Input: part model. Units: mm. Frame: model coordinates. Face numbers are marked on the shaded views. A direction names the side the tool comes from. Give positions to 0.01 mm unless a question says otherwise; leave off trailing zeros. Loops run counter-clockwise (first coordinate to the right, second up) from the corner with the lowest first, then second, coordinate; pieces in that order, holes last.
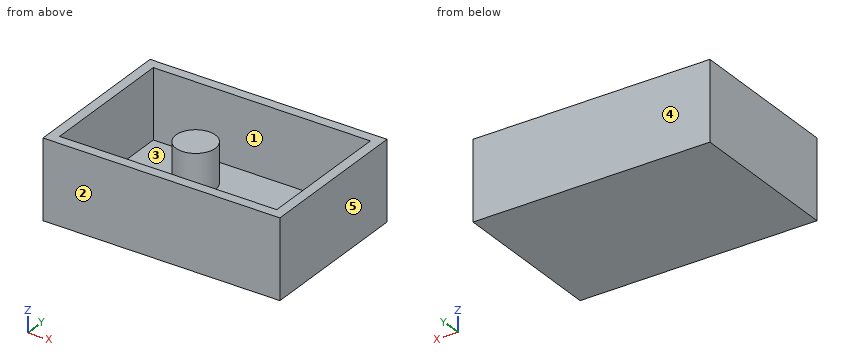
from build123d import *

# Parameters (mm, degrees)
F0_W     = 152.4
F0_H     = 101.6
F1_DEPTH = 50.8
F2_T     = -6.35
F3_R     = 12.7
F4_DEPTH = 25.4


with BuildPart() as f1:
    # F0 (on Top) → F1 (new body)
    with BuildSketch(Plane.XY):
        Rectangle(F0_W, F0_H)
    extrude(amount=F1_DEPTH)

    # F2
    f2_openings = [f1.faces().sort_by_distance(p)[0] for p in [
        (0, 0, 50.8),
    ]]
    offset(amount=F2_T, openings=f2_openings)

    # F3 (on face) → F4 (join)
    with BuildSketch(Plane.XY.offset(6.35)):
        with Locations((-25.4, 19.05)):
            Circle(F3_R)
    extrude(amount=F4_DEPTH)


solid = f1.part
(1) Ray query, probe 1 along Y at (x, z) = (64, 33.5); probe 2 along X at (y, z) = (-32.5, 36.5); probe 3 along X at (y, z) = (23.5, 9). Return the intervals inside material, ascending.
Values follow:
probe 1: y = -50.8 to -44.45, 44.45 to 50.8
probe 2: x = -76.2 to -69.85, 69.85 to 76.2
probe 3: x = -76.2 to -69.85, -37.29 to -13.51, 69.85 to 76.2
(2) Cut plane C-C (x = -2). Return the cut outline in (y, z).
Values follow:
outline: (-50.8, 0) - (50.8, 0) - (50.8, 50.8) - (44.45, 50.8) - (44.45, 6.35) - (-44.45, 6.35) - (-44.45, 50.8) - (-50.8, 50.8) - close
(3) Mould query, pull axis Y, two halves, no side actions, for the marked faces 3, 4 and 5. Classes: +Y half, -Y half, draft (parallel to the pull), parting line (faces both ways), or undercut.
Values follow:
face 3: undercut
face 4: +Y half
face 5: draft
(4) Cut plane B-B (z = 43.5). Return the cut outline in (x, y).
Values follow:
outline: (-76.2, -50.8) - (76.2, -50.8) - (76.2, 50.8) - (-76.2, 50.8) - close; hole (-69.85, -44.45) - (69.85, -44.45) - (69.85, 44.45) - (-69.85, 44.45) - close
(5) Pin query (flat end, axial travel): pin 1 Ø12.5 at (x, y) = (-20, 14.5) entering from +Z; pin 2 Ø6 at (x, y) = (60.5, 31.5) entering from -Z; pin 3 Ø2 at (x, y) = (-52, 29) entering from +Z. Return the tip coordinate at first contact, or that it passes through.
Values follow:
pin 1: stops at z = 31.75
pin 2: stops at z = 0
pin 3: stops at z = 6.35
(6) Cut plane A-A (z = 26). Return the cut outline in (x, y).
Values follow:
outline: (-76.2, -50.8) - (76.2, -50.8) - (76.2, 50.8) - (-76.2, 50.8) - close; circle Ø25.4 at (-25.4, 19.05); hole (-69.85, -44.45) - (69.85, -44.45) - (69.85, 44.45) - (-69.85, 44.45) - close
(7) Cut plane D-D (y = -32). Return the cut outline in (x, z), and give its area (3 significant figures).
Values follow:
outline: (-76.2, 0) - (76.2, 0) - (76.2, 50.8) - (69.85, 50.8) - (69.85, 6.35) - (-69.85, 6.35) - (-69.85, 50.8) - (-76.2, 50.8) - close
area: 1,530 mm2
(8) Reachability of the marked faces 1 and 2 from +Z, -Z, +X, -X, +Y, -Y: full face, straight path, thin tool, end or side. Return the list, or none.
Values follow:
face 1: +Z
face 2: +Z, -Z, +X, -X, -Y
